The model under review builds one solid part; all positions refer to its coordinate system, in mm. Coordinates: 2 decimals unless noted, no trailing zeros. Write each loop counter-clockwise with the first axis right and the second up, starting at its lowest first coordinate (ties: lowest second). Pieces come first, ordered by that corner, then holes.
1) Add section B-B, the plane y = 6.35. State the section outline as (x, z) points (3 decimals).
2) Add section C-C, the plane x = 3.5. State the section outline as (y, z) points.
3) For line 1 (X direction, y = 6, z = 4); line 2 (X direction, y = 4.75, z = -5.5); line 3 (X direction, y = 4.5, z = -0.75), list the stretches that pass through material, from the lowest coordinate up.
4) Mouldability with a two-part tool opening along Z and no side actions: class faces 1 (the flat face through (31.75, 6, 0)), 2 (the flat face through (16, 6, -6.35)), 3 (the cylindrical face through (14.015, 6.439, -0.413)) as released by +Z, released by -Z, zero draft, split by the parting line, or undercut.
5) Add section D-D, the plane z = 4.75. State the section outline as (x, y) points, then the cut area to 3 significant figures.
6) Add section A-A, the plane z = 0. State the section outline as (x, y) points, then the cut area to 3 significant figures.
from build123d import *

# Parameters (mm, degrees)
SKETCH1_W           = 31.75
SKETCH1_H           = 12.7
BOSS_EXTRUDE1_DEPTH = 6.35
SKETCH2_R           = 2.0193
CUT_EXTRUDE1_DEPTH  = 37.477972806
SKETCH3_R           = 1.905
CUT_EXTRUDE2_DEPTH  = 35.780382402


with BuildPart() as part:
    # Sketch1 → Boss-Extrude1 (new, symmetric)
    with BuildSketch(Plane.XY):
        with Locations((15.875, 6.35)):
            Rectangle(SKETCH1_W, SKETCH1_H)
    extrude(amount=BOSS_EXTRUDE1_DEPTH, both=True)

    # Sketch2 → Cut-Extrude1 (cut, through all)
    with BuildSketch(Plane.XY.offset(6.35)):
        with Locations((4.7625, 6.35)):
            Circle(SKETCH2_R)
        with Locations((26.9875, 6.35)):
            Circle(SKETCH2_R)
    extrude(amount=-CUT_EXTRUDE1_DEPTH, mode=Mode.SUBTRACT)

    # Sketch3 → Cut-Extrude2 (cut, through all)
    with BuildSketch(Plane(origin=(0, 12.7, 0), x_dir=(1, 0, 0), z_dir=(0, 1, 0))):
        with Locations(Location((15.875, 0, 0), (0, 0, 270))):
            Circle(SKETCH3_R)
    extrude(amount=-CUT_EXTRUDE2_DEPTH, mode=Mode.SUBTRACT)


solid = part.part
Geometry results:
1. outline: (0, -6.35) - (2.743, -6.35) - (2.743, 6.35) - (0, 6.35) - close; (6.782, -6.35) - (24.968, -6.35) - (24.968, 6.35) - (6.782, 6.35) - close; (29.007, -6.35) - (31.75, -6.35) - (31.75, 6.35) - (29.007, 6.35) - close; hole circle Ø3.81 at (15.875, 0)
2. outline: (0, -6.35) - (4.77, -6.35) - (4.77, 6.35) - (0, 6.35) - close; (7.93, -6.35) - (12.7, -6.35) - (12.7, 6.35) - (7.93, 6.35) - close
3. line 1: x = 0 to 2.77, 6.75 to 25, 28.98 to 31.75
3. line 2: x = 0 to 3.53, 5.99 to 25.76, 28.22 to 31.75
3. line 3: x = 0 to 3.95, 5.57 to 14.12, 17.63 to 26.18, 27.8 to 31.75
4. face 1: zero draft
4. face 2: released by -Z
4. face 3: undercut
5. outline: (0, 0) - (31.75, 0) - (31.75, 12.7) - (0, 12.7) - close; hole circle Ø4.04 at (4.76, 6.35); hole circle Ø4.04 at (26.99, 6.35)
5. area: 378 mm2
6. outline: (0, 0) - (13.97, 0) - (13.97, 12.7) - (0, 12.7) - close; (17.78, 0) - (31.75, 0) - (31.75, 12.7) - (17.78, 12.7) - close; hole circle Ø4.04 at (4.76, 6.35); hole circle Ø4.04 at (26.99, 6.35)
6. area: 329 mm2
